Can you work these out from the model? Positions are in its coordinate system, mm. Face numbers are marked on the shaded views. A direction names the side the tool comes from. Give positions to 0.01 mm unless a question says otherwise; leave off trailing zeros. Loops run counter-clockwise (first coordinate to the right, second up) from the corner with the lowest first, then second, coordinate; pieces in that order, holes last. Notation, with made-up numbers: (-6.5, -10.5) - (16.5, -10.5) arc R29 ccw to (16.5, 19.5) - close; hole circle Ø8 at (87, 32). An arc over 180 degrees is marked (long way). Answer in a Markdown table with one row per item.
from build123d import *

# Parameters (mm, degrees)
SKETCH_1_R          = 6
SKETCH_1_R_2        = 3
EXTRUDE_1_DEPTH     = 9.5
CHAMFER_1_SIZE      = 0.5
SKETCH_2_R          = 5.5
CUT_EXTRUDE_1_DEPTH = 0.5


with BuildPart() as part:
    # 스케치1 → 보스-돌출1 (new, symmetric)
    with BuildSketch(Plane.XY):
        Circle(SKETCH_1_R)
        Circle(SKETCH_1_R_2, mode=Mode.SUBTRACT)
    extrude(amount=EXTRUDE_1_DEPTH, both=True)

    # 모따기1
    chamfer_1_edges = [part.edges().sort_by_distance(p)[0] for p in [
        (-6, 0, -9.5),
        (-6, 0, 9.5),
    ]]
    chamfer(chamfer_1_edges, length=CHAMFER_1_SIZE)

    # 스케치2 → 컷-돌출1 (cut)
    with BuildSketch(Plane.XY.offset(9.5)):
        Circle(SKETCH_2_R)
    cut_extrude_1 = extrude(amount=-CUT_EXTRUDE_1_DEPTH, mode=Mode.SUBTRACT)

    # 대칭 복사1: 컷-돌출1 across plane
    add(cut_extrude_1.mirror(Plane.XY), mode=Mode.SUBTRACT)

    # 스케치3 → 컷-회전1 (revolve, cut)
    with BuildSketch(Plane(origin=(0, 0, 0), x_dir=(0, 0, -1), z_dir=(1, 0, 0)), mode=Mode.PRIVATE) as cut_revolve_1_sk:
        Polygon((-4.625, 6), (-5.125, 6), (-4.875, 5.566987298), align=None)
        Polygon((4.625, 6), (5.125, 6), (4.875, 5.566987298), align=None)
    revolve(cut_revolve_1_sk.sketch.rotate(Axis((0, 0, 9), (0, 0, -1)), 180), axis=Axis((0, 0, 9), (0, 0, -1)), mode=Mode.SUBTRACT)


solid = part.part
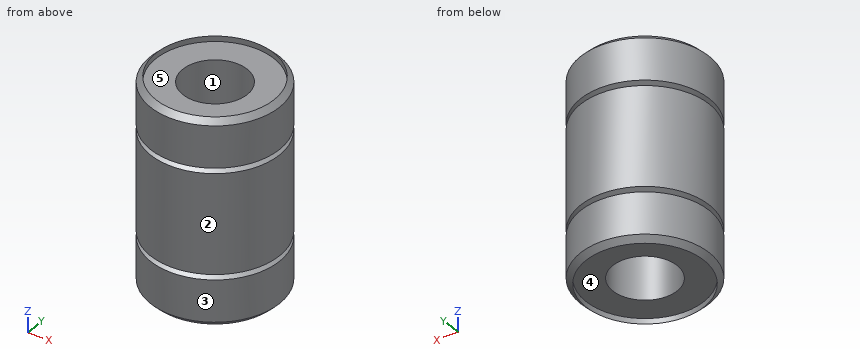
Q1. For pin 1 (5.5 mm diameter, centred on x = 0, y = 0, fed in from +Z); pin 2 (3.5 mm diameter, centred on x = 2.5, y = -2, fed in from -Z); pin 3 (4 mm diameter, centred on x = -3, z = -3, fed in from +Y); pin 4 (1 mm diameter, centred on x = 0.5, z = -3.5, fed in from -Y), each with a flat end and sliding along its axis, tell me the tip position at first contact or that it passes through.
Checked values:
| item | result |
|---|---|
| pin 1 | passes through |
| pin 2 | stops at z = -9 |
| pin 3 | stops at y = 5.92 |
| pin 4 | stops at y = -6 |
Q2. If I drill on line 1 (X direction, y = 0, z = 1.75); line 2 (Z direction, x = -3.75, y = 2.5); line 3 (Y direction, x = 2.5, z = 5.75), over which ranges is the centre line in solid material (lowest first)? Write a range as [from, to].
Checked values:
| item | result |
|---|---|
| line 1 | x = [-6, -3], [3, 6] |
| line 2 | z = [-9, 9] |
| line 3 | y = [-5.45, -1.66], [1.66, 5.45] |
Q3. Imagine slicing it at A-A, the plane x = 0. Write out the boundary of the cut face in (y, z) (3 decimals).
Checked values:
| item | result |
|---|---|
| outline | (-6, -9) - (-5.5, -9.5) - (-5.5, -9) - (-3, -9) - (-3, 9) - (-5.5, 9) - (-5.5, 9.5) - (-6, 9) - (-6, 5.125) - (-5.567, 4.875) - (-6, 4.625) - (-6, -4.625) - (-5.567, -4.875) - (-6, -5.125) - close; (3, -9) - (5.5, -9) - (5.5, -9.5) - (6, -9) - (6, -5.125) - (5.567, -4.875) - (6, -4.625) - (6, 4.625) - (5.567, 4.875) - (6, 5.125) - (6, 9) - (5.5, 9.5) - (5.5, 9) - (3, 9) - close |
Q4. On a 3-axis mill with a long thin cutter (end or side, diameter ignored), from which of +Z, -Z, +X, -X, +Y, -Y can I reach the whole of each face in a straight line? I mean the marked faces 3, 4 and 5. Say none if no direction works.
Checked values:
| item | result |
|---|---|
| face 3 | +Z, -Z |
| face 4 | -Z |
| face 5 | +Z |
Q5. If we mould it in two halves opening along Y, with no side actions, what happens to the marked faces 1 and 2? For each: released by +Y, released by -Y, zero draft, split by the parting line, or undercut.
Checked values:
| item | result |
|---|---|
| face 1 | undercut |
| face 2 | split by the parting line |
Q6. Imagine slicing it at C-C, the plane z = -6.5. Write out the boundary of the cut face in (x, y).
Checked values:
| item | result |
|---|---|
| outline | circle Ø12 at (0, 0); hole circle Ø6 at (0, 0) |
